Here's how the part is built. I have some questions about the finished solid (model axes, mm). Coordinates: 2 decimals unless noted, no trailing zeros. Write each loop counter-clockwise with the first axis right and the second up, starting at its lowest first coordinate (ties: lowest second). Pieces come first, ordered by that corner, then holes. Notation, with made-up numbers: (23.25, 4) -> (51.25, 4) arc R29 ccw to (51.25, 34) -> close; hole circle Ø10 at (-39.5, -16.5). An arc over 180 degrees is marked (long way). Use CSV: the item, a comma, the result in double quotes. Start each with the question number.
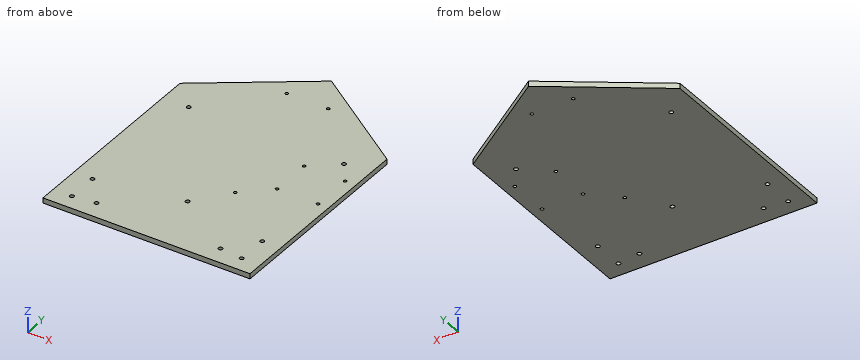
```python
from build123d import *

# Parameters (mm, degrees)
SKETCH1_R           = 2
SKETCH1_R_2         = 1.5
BOSS_EXTRUDE1_DEPTH = 5


with BuildPart() as part:
    # Sketch1 → Boss-Extrude1 (new body)
    with BuildSketch(Plane.XY):
        Polygon((-92.496965253, 104.871794872), (-92.496965253, -95.128205128), (107.503034747, -95.128205128), (107.503034747, 104.871794872), (7.503034747, 174.871794872), align=None)
        with Locations((89.503034747, -80.128205128)):
            Circle(SKETCH1_R, mode=Mode.SUBTRACT)
        with Locations((-74.496965253, -80.128205128)):
            Circle(SKETCH1_R, mode=Mode.SUBTRACT)
        with Locations((27.503034747, 139.871794872)):
            Circle(SKETCH1_R_2, mode=Mode.SUBTRACT)
        with Locations((-12.496965253, 139.871794872)):
            Circle(SKETCH1_R_2, mode=Mode.SUBTRACT)
        with Locations((89.503034747, -50.128205128)):
            Circle(SKETCH1_R, mode=Mode.SUBTRACT)
        with Locations((-74.496965253, -50.128205128)):
            Circle(SKETCH1_R, mode=Mode.SUBTRACT)
        with Locations((7.503034747, -35.128205128)):
            Circle(SKETCH1_R, mode=Mode.SUBTRACT)
        with Locations((32.403034747, -3.128205128)):
            Circle(SKETCH1_R_2, mode=Mode.SUBTRACT)
        with Locations((57.503034747, 19.871794872)):
            Circle(SKETCH1_R_2, mode=Mode.SUBTRACT)
        with Locations((-52.496965253, -77.628205128)):
            Circle(SKETCH1_R, mode=Mode.SUBTRACT)
        with Locations((67.503034747, -77.628205128)):
            Circle(SKETCH1_R, mode=Mode.SUBTRACT)
        with Locations((-67.496965253, 79.871794872)):
            Circle(SKETCH1_R, mode=Mode.SUBTRACT)
        with Locations((82.503034747, 79.871794872)):
            Circle(SKETCH1_R, mode=Mode.SUBTRACT)
        with Locations((57.503034747, 59.471794872)):
            Circle(SKETCH1_R_2, mode=Mode.SUBTRACT)
        with Locations((97.103034747, 19.871794872)):
            Circle(SKETCH1_R_2, mode=Mode.SUBTRACT)
        with Locations((97.103034747, 59.471794872)):
            Circle(SKETCH1_R_2, mode=Mode.SUBTRACT)
    extrude(amount=BOSS_EXTRUDE1_DEPTH)


solid = part.part
```
Item 1: If I drill on line 1 along Y through (x, z) = (-73.5, 1.95); line 2 along Y through (x, z) = (90, 2.4); line 3 along X through (y, z) = (20.5, 3.45), over which ranges is the centre line in solid material (lowest first)?
Item 2: I want a section at B-B on x = -20. Please give me the cut outline in (y, z), then the cut area to 3 significant figures.
Item 3: I want a section at C-C on x = 74. Please give me the cut outline in (y, z).
Item 4: I want a section at A-A on z = 2.8. Count the separate pieces of the cut face and the enclosed holes in it, then the cut area to 3 significant figures.
Item 5: I'm going to push flat-ended pins straight in: pin 1 (3 mm diameter, centred on x = 7.5, y = -35.13, fed in from +Z); pin 2 (3 mm diameter, centred on x = -42.5, z = 1, fed in from +Y); pin 3 (1 mm diameter, centred on x = 14.5, z = 4, fed in from +Y). Where does each tip first touch, or does it pass through?
Geometry says:
1,line 1,"-95.13 to -81.86, -78.39 to -51.86, -48.39 to 118.17"
1,line 2,"-95.13 to -82.07, -78.19 to -52.07, -48.19 to 117.12"
1,line 3,"-92.5 to 56.14, 58.87 to 95.74, 98.47 to 107.5"
2,outline,"(-95.13, 0) -> (155.62, 0) -> (155.62, 5) -> (-95.13, 5) -> close"
2,area,"1,250 mm2"
3,outline,"(-95.13, 0) -> (128.32, 0) -> (128.32, 5) -> (-95.13, 5) -> close"
4,separate pieces,"1"
4,enclosed holes,"16"
4,area,"46,800 mm2"
5,pin 1,"through"
5,pin 2,"y = 140.92"
5,pin 3,"y = 170.32"
